Part model, mm, in its own coordinate system. Face numbers are marked on the shaded views. A direction names the side the tool comes from. Round coordinates to 2 decimals unless told otherwise and drop trailing zeros. Loops run counter-clockwise (first coordinate to the right, second up) from the corner with the lowest first, then second, coordinate; pieces in that order, holes last. Notation, with made-up numbers: (-5.5, 79) -> (29.5, 79) arc R38 ccw to (29.5, 118) -> close; hole circle Ø6 at (-4.5, 13). An arc over 180 degrees is marked (long way). Answer as CSV lines item,"result".
Solid Edge part; units mm, degrees
sketch "Sketch1" plane through (0, 0, 0) normal (0, 0, 1) x (1, 0, 0)
  circle A0 centre (0, 0) radius 2.29
extrude "Protrusion1" add sketch "Sketch1" along normal blind 6
sketch "Sketch2" plane through (0, 0, 0) normal (0, -1, 0) x (1, 0, 0)
  spline S0 degree 3 poles (1.7792, 6.15) (2.5889, 8.2091) (0.8279, 9.3298) (0, 9.56) knots 0 0 0 0 1 1 1 1
  line L0 (0, 6.15) -> (0, 9.56)
  line L1 (0, 6.15) -> (1.7792, 6.15)
revolve "RevolvedProtrusion1" add sketch "Sketch2" angle 360 about axis through (0, 0, 5.85) along (0, 0, 1)
sketch "Sketch3" plane through (0, 0, 6.9992) normal (0, 0, 1) x (1, 0, 0)
  line L0 (-4.048, -9.105) -> (0.0835, -4.7436)
  line L1 (-5.4114, -8.3178) -> (-4.048, -9.105)
  line L2 (-1.2964, -1.1905) -> (-5.4114, -8.3178)
  arc A0 (0.1991, -1.7487) -> (-1.2964, -1.1905) centre (0, 0) cw
  line L3 (0.0835, -4.7436) -> (0.1991, -1.7487)
  line L4 (1.6791, -0.5274) -> (9.9091, -0.5274)
  line L5 (9.9091, -0.5274) -> (9.9091, 1.0468)
  line L6 (9.9091, 1.0468) -> (4.0663, 2.4441)
  line L7 (4.0663, 2.4441) -> (1.4149, 1.0468)
  arc A1 (1.4149, 1.0468) -> (1.6791, -0.5274) centre (0, 0) cw
extrude "ExtrudedProtrusion_6" add sketch "Sketch3" along normal blind 0.15
sketch "Sketch4" plane through (0, 0, 6.9992) normal (0, 0, 1) x (1, 0, 0)
  line L0 (-5.8611, 8.0582) -> (-4.1498, 2.2995)
  line L1 (-4.1498, 2.2995) -> (-1.614, 0.702)
  arc A0 (-1.614, 0.702) -> (-0.3828, 1.7179) centre (0, 0) cw
  line L2 (-0.3828, 1.7179) -> (-4.4978, 8.8453)
  line L3 (-4.4978, 8.8453) -> (-5.8611, 8.0582)
extrude "ExtrudedProtrusion_7" add sketch "Sketch4" against normal blind 0.15
sketch "Sketch5" plane through (0, 0, 6) normal (0, 0, 1) x (-1, 0, 0)
  circle A0 centre (0, 0) radius 1.2
extrude "ExtrudedCutout_2" cut sketch "Sketch5" against normal blind 5.2864
sketch "Sketch6" plane through (0, 0, 6.15) normal (0, 0, -1) x (1, 0, 0)
  circle A0 centre (0, 0) radius 0.536
extrude "Protrusion2" add sketch "Sketch6" along normal up to vertex (6.15 mm away)
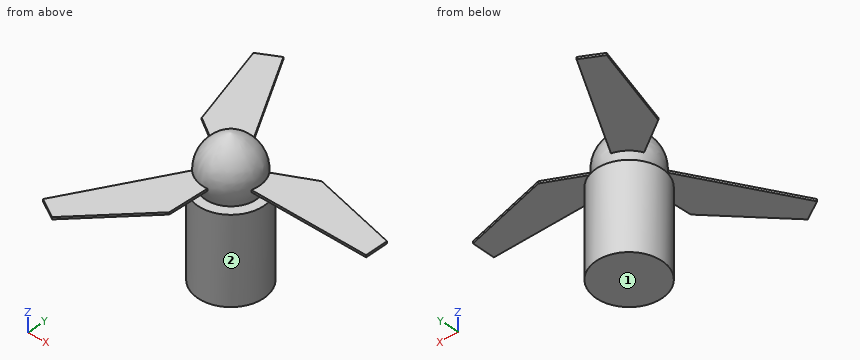
Q1. Saw through at B-B, the plane x = 7. Write the cut outline in (y, z).
Geometry results:
outline,"(-0.53, 7) -> (1.74, 7) -> (1.74, 7.15) -> (-0.53, 7.15) -> close"
Q2. Which spindle directions (+Z, -Z, +X, -X, +Y, -Y) get a long thin tool onto all of the face, cutting with end or side? Do the marked faces 1 and 2. Say none if no direction does.
Geometry results:
face 1,"-Z, +X, -X, +Y, -Y"
face 2,"-Z"
Q3. Drill centre lines: line 1 along Y through (x, z) = (0, 2); line 2 along Z through (x, y) = (-3.75, 6); line 3 along Z through (x, y) = (3, 0.25). Where is each one in solid material? Low to high.
Geometry results:
line 1,"-2.29 to -1.2, -0.54 to 0.54, 1.2 to 2.29"
line 2,"6.85 to 7"
line 3,"7 to 7.15"
Q4. Saw through at A-A, the plane z = 2.25. Write the cut outline in (x, y).
Geometry results:
outline,"circle Ø4.58 at (0, 0); circle Ø1.07 at (0, 0); hole circle Ø2.4 at (0, 0)"
Q5. Saw through at C-C, the plane y = 5.5. Write the cut outline in (x, z).
Geometry results:
outline,"(-5.1, 6.85) -> (-2.57, 6.85) -> (-2.57, 7) -> (-5.1, 7) -> close"
Q6. Drop flat-ended pins along their axis: P1, Ø1.5, axis at y = 0.5, z = 3.5, coming from the -X side; P2, Ø2, axis at x = 2.5, y = -2, coming from the +Z side; P3, Ø6, axis at x = -4, y = 4.5, coming from the -Z side. Give the stop position or say it passes through.
Geometry results:
P1,"x = -2.29"
P2,"z = 6"
P3,"z = 6.85"
